The listing builds one solid part. Answer for the finished solid, in the listing's coordinates (mm). Face numbers are marked on the shaded views. A direction names the side the tool comes from. Round coordinates to 2 decimals unless told otherwise and drop trailing zeros. Write each loop counter-clockwise with the first axis right and the second up, starting at its lowest first coordinate (ties: lowest second). Pieces come first, ordered by that corner, then holes. Notation, with made-up numbers: (-37.5, 88.25) -> (-11.5, 88.25) arc R19 ccw to (-11.5, 125.25) -> close; hole circle Ø8 at (-27, 25). An arc over 180 degrees is marked (long way). Write each question's results on one line, items separated by ' | '. Start each with the question number.
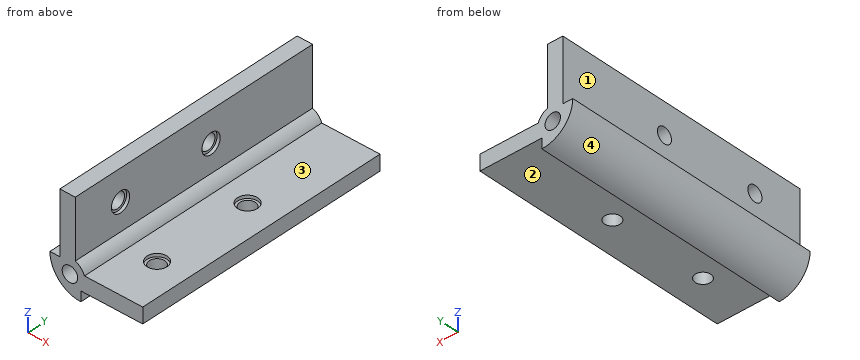
```python
from build123d import *

# Parameters (mm, degrees)
SKETCH4_R           = 2.5
BOSS_EXTRUDE1_DEPTH = 64.27
SKETCH5_R           = 2.5
CUT_EXTRUDE1_DEPTH  = 72.548291037
SKETCH6_R           = 2.5
CUT_EXTRUDE2_DEPTH  = 74.179063133
SKETCH7_R           = 3.25
CUT_EXTRUDE3_DEPTH  = 1
SKETCH8_R           = 3.25
CUT_EXTRUDE4_DEPTH  = 1
SKETCH9_R           = 2.5
BOSS_EXTRUDE2_DEPTH = 20


with BuildPart() as part:
    # Sketch4 → Boss-Extrude1 (new body)
    with BuildSketch(Plane(origin=(0, 0, 0), x_dir=(1, 0, 0), z_dir=(0, 1, 0))):
        with BuildLine():
            Line((-5.286754077, 14.301163994), (13.559651759, 14.301163994))
            Line((13.559651759, 14.301163994), (13.559651759, 19.301163994))
            Line((13.559651759, 19.301163994), (-6.440348241, 19.301163994))
            Line((-6.440348241, 19.301163994), (-6.440348241, 22.501163994))
            ThreePointArc((-6.440348241, 22.501163994), (-13.511416053, 19.572231806), (-16.440348241, 12.501163994))
            Line((-16.440348241, 12.501163994), (-13.240348241, 12.501163994))
            Line((-13.240348241, 12.501163994), (-13.240348241, -7.498836006))
            Line((-13.240348241, -7.498836006), (-8.240348241, -7.498836006))
            Line((-8.240348241, -7.498836006), (-8.240348241, 11.347569829))
            ThreePointArc((-8.240348241, 11.347569829), (-6.440348241, 12.501163994), (-5.286754077, 14.301163994))
        make_face()
        with Locations(Location((-9.975882147, 16.0366979, 0), (0, 0, 270))):
            Circle(SKETCH4_R, mode=Mode.SUBTRACT)
    extrude(amount=BOSS_EXTRUDE1_DEPTH)

    # Sketch5 → Cut-Extrude1 (cut, through all)
    with BuildSketch(Plane(origin=(0, 0, -19.301163994), x_dir=(-1, 0, 0), z_dir=(0, 0, -1))):
        with Locations((-3.559651759, 48.2025)):
            Circle(SKETCH5_R)
        with Locations((-3.559651759, 16.0675)):
            Circle(SKETCH5_R)
    extrude(amount=-CUT_EXTRUDE1_DEPTH, mode=Mode.SUBTRACT)

    # Sketch6 → Cut-Extrude2 (cut, through all)
    with BuildSketch(Plane.ZY.offset(13.240348241)):
        with Locations((-2.501163994, 48.2025)):
            Circle(SKETCH6_R)
        with Locations((-2.501163994, 16.0675)):
            Circle(SKETCH6_R)
    extrude(amount=-CUT_EXTRUDE2_DEPTH, mode=Mode.SUBTRACT)

    # Sketch7 → Cut-Extrude3 (cut)
    with BuildSketch(Plane(origin=(-8.240348241, 0, 0), x_dir=(0, 0, -1), z_dir=(1, 0, 0))):
        with Locations((2.501163994, 48.2025)):
            Circle(SKETCH7_R)
        with Locations((2.501163994, 16.0675)):
            Circle(SKETCH7_R)
    extrude(amount=-CUT_EXTRUDE3_DEPTH, mode=Mode.SUBTRACT)

    # Sketch8 → Cut-Extrude4 (cut)
    with BuildSketch(Plane.XY.offset(-14.301163994)):
        with Locations((3.559651759, 48.2025)):
            Circle(SKETCH8_R)
        with Locations((3.559651759, 16.0675)):
            Circle(SKETCH8_R)
    extrude(amount=-CUT_EXTRUDE4_DEPTH, mode=Mode.SUBTRACT)

    # Sketch9 → Boss-Extrude2 (add)
    with BuildSketch(Plane(origin=(0, 64.27, 0), x_dir=(1, 0, 0), z_dir=(0, 1, 0))):
        with BuildLine():
            Line((-6.440348241, 22.501163994), (-6.440348241, 19.301163994))
            Line((-6.440348241, 19.301163994), (13.559651759, 19.301163994))
            Line((13.559651759, 19.301163994), (13.559651759, 14.301163994))
            Line((13.559651759, 14.301163994), (-5.286754077, 14.301163994))
            ThreePointArc((-5.286754077, 14.301163994), (-6.440348241, 12.501163994), (-8.240348241, 11.347569829))
            Line((-8.240348241, 11.347569829), (-8.240348241, -7.498836006))
            Line((-8.240348241, -7.498836006), (-13.240348241, -7.498836006))
            Line((-13.240348241, -7.498836006), (-13.240348241, 12.501163994))
            Line((-13.240348241, 12.501163994), (-16.440348241, 12.501163994))
            ThreePointArc((-16.440348241, 12.501163994), (-13.511416053, 19.572231806), (-6.440348241, 22.501163994))
        make_face()
        with Locations(Location((-9.975882147, 16.0366979, 0), (0, 0, 270))):
            Circle(SKETCH9_R, mode=Mode.SUBTRACT)
    extrude(amount=BOSS_EXTRUDE2_DEPTH)


solid = part.part
```
Q1. Each of these flat-tipped pins is pushed along its axis until it touches: pin 1 (8.5 mm diameter, centred on x = 3.56, y = 48.2, fed in from -Z); pin 2 (10 mm diameter, centred on x = -12, y = 44, fed in from -Z); pin 3 (4 mm diameter, centred on y = 28, z = -10.5, fed in from +X); pin 4 (6 mm diameter, centred on x = -2.5, z = 0, fed in from -Y). Where does it stop, or does it pass through?
Q2. Find the intervals of material crossed by line 1 (Y direction, x = 4.75, z = -16.5); line 2 (X direction, y = 18, z = 6); line 3 (Z direction, x = -3, y = 24), in increasing order.
Q3. The part is cut by section A-A, the plane z = -1. Write down the section's boundary in (x, y).
Q4. The part is cut by section D-D, the plane z = 4. Write down the section's boundary in (x, y), then the cut area to 3 significant figures.
Q5. The part is cut by section C-C, the plane y = 30.5. Write down the section's boundary in (x, z).
Q6. For the marked faces 1, 2, 3 and 4, determine the directions among +Z, -Z, +X, -X, +Y, -Y from which every point of the face is accessible in a straight line to the end or side of a thin tool.
Q7. The part is cut by section B-B, the plane x = 2. Write down the section's boundary in (y, z).
Answers follow:
1) pin 1: z = -19.3 | pin 2: z = -22.49 | pin 3: x = -6.44 | pin 4: through
2) line 1: 0 to 13.87, 18.27 to 46, 50.4 to 84.27 | line 2: -13.24 to -8.24 | line 3: -19.3 to -14.3
3) outline: (-13.24, 0) -> (-8.24, 0) -> (-8.24, 13.18) -> (-9.24, 13.18) -> (-9.24, 14.07) -> (-13.24, 14.07) -> close; (-13.24, 18.07) -> (-9.24, 18.07) -> (-9.24, 18.95) -> (-8.24, 18.95) -> (-8.24, 45.32) -> (-9.24, 45.32) -> (-9.24, 46.2) -> (-13.24, 46.2) -> close; (-13.24, 50.2) -> (-9.24, 50.2) -> (-9.24, 51.09) -> (-8.24, 51.09) -> (-8.24, 84.27) -> (-13.24, 84.27) -> close
4) outline: (-13.24, 0) -> (-8.24, 0) -> (-8.24, 84.27) -> (-13.24, 84.27) -> close | area: 421 mm^2
5) outline: (-16.44, -12.5) arc R10 ccw to (-6.44, -22.5) -> (-6.44, -19.3) -> (13.56, -19.3) -> (13.56, -14.3) -> (-5.29, -14.3) arc R5 ccw to (-8.24, -11.35) -> (-8.24, 7.5) -> (-13.24, 7.5) -> (-13.24, -12.5) -> close; hole circle Ø5 at (-9.98, -16.04)
6) face 1: +Z, -X, +Y, -Y | face 2: -Z, +X, +Y, -Y | face 3: +Z, +X, +Y, -Y | face 4: -Z, -X, +Y, -Y
7) outline: (0, -19.3) -> (14.11, -19.3) -> (14.11, -15.3) -> (13.22, -15.3) -> (13.22, -14.3) -> (0, -14.3) -> close; (18.02, -19.3) -> (46.25, -19.3) -> (46.25, -15.3) -> (45.35, -15.3) -> (45.35, -14.3) -> (18.92, -14.3) -> (18.92, -15.3) -> (18.02, -15.3) -> close; (50.16, -19.3) -> (84.27, -19.3) -> (84.27, -14.3) -> (51.05, -14.3) -> (51.05, -15.3) -> (50.16, -15.3) -> close
